Autodesk Inventor part; units mm, degrees
ref_plane "YZ Plane" through (0, 0, 0) normal (1, 0, 0) x (0, 1, 0)
ref_plane "XZ Plane" through (0, 0, 0) normal (0, 1, 0) x (-1, 0, 0)
ref_plane "XY Plane" through (0, 0, 0) normal (0, 0, 1) x (1, 0, 0)
sketch "Sketch1" plane through (0, 0, 0) normal (0, 0, 1) x (1, 0, 0)
  line L0 (0, 0) -> (51, 0)
  line L1 (51, 0) -> (51, 90)
  line L2 (51, 90) -> (0, 90)
  line L3 (0, 90) -> (0, 0)
  dimension "d0" = 51
  dimension "d1" = 90
extrude "Extrusion1" add sketch "Sketch1" along normal blind 5
sketch "Sketch2" plane through (0, 0, 5) normal (0, 0, 1) x (1, 0, 0)
  line L0 (0, 0) -> (51, 0) construction
  line L1 (25.5, 0) -> (25.5, 90) construction
  line L2 (51, 90) -> (0, 90) construction
  line L3 (51, 0) -> (51, 90) construction
  line L4 (51, 45) -> (0, 45) construction
  line L5 (25.5, 45) -> (25.5, 35) construction
  line L6 (25.5, 35) -> (18, 35) construction
  line L7 (18, 35) -> (18, 50) construction
  line L8 (18, 50) -> (33, 50) construction
  line L9 (33, 50) -> (33, 35) construction
  dimension "d23" = 10
  dimension "d24" = 7.5
  dimension "d25" = 15
  dimension "d26" = 15
sketch "Sketch3" plane through (0, 0, 0) normal (0, 0, -1) x (-1, 0, 0)
  line L0 (-51, 90) -> (0, 90)
  line L1 (-51, 90) -> (-41, 90)
  line L2 (-41, 90) -> (-41, 0)
  line L3 (0, 90) -> (-10.0159, 90)
  line L4 (-10.0159, 90) -> (-10.0159, 0)
  line L5 (0, 0) -> (-51, 0)
  line L6 (-51, 90) -> (-51, 79)
  line L7 (-51, 79) -> (0, 79)
  line L8 (-51, 0) -> (-51, 8)
  line L9 (-51, 0) -> (-51, 90)
  line L10 (-51, 8) -> (0, 8)
  line L11 (-51, 90) -> (-46, 90)
  line L12 (-51, 79) -> (-46, 79)
  line L13 (-46, 90) -> (-46, 69)
  line L14 (-10.0159, 45) -> (-4.0159, 45)
  line L15 (0, 90) -> (0, 0)
  line L16 (-41, 90) -> (-41, 48.5) construction
  line L17 (-47, 45) -> (-4.0159, 45)
  line L18 (-47, 43.5703) -> (-3.108, 43.5703)
  line L19 (-41, 90) -> (-47, 90)
  line L20 (-47, 90) -> (-47, 0)
  line L21 (-47, 0) -> (-47, 18)
  line L22 (-10.0159, 0) -> (-4.0159, 0)
  line L23 (-4.0159, 0) -> (-4.0159, 18)
  line L24 (-10.0159, 90) -> (-4.0159, 90)
  line L25 (-4.0159, 90) -> (-4.0159, 69)
  point P0 (-5, 69)
  point P1 (-46, 18)
  point P2 (-5, 18)
  point P3 (-48.5, 90)
  point P4 (-25.054, 43.5703)
  point P5 (-25.508, 45)
  point P6 (-47, 69)
  point P7 (-4.0159, 43.5703)
  dimension "d8" = 11
  dimension "d9" = 8
  dimension "d15" = 21
  dimension "d38" = 5
  dimension "d41" = 6
  dimension "d47" = 10
  dimension "d48" = 10.016
  dimension "d50" = 1.5
  dimension "d54" = 6
  dimension "d55" = 18
  dimension "d56" = 6
  dimension "d57" = 6
hole "Hole1" at (4.0159, 69, 0) at (4.0159, 43.5703, 0) at (4.0159, 18, 0) at (47, 18, 0) at (47, 43.5703, 0) at (47, 69, 0) direction (0, 0, 1) diameter 2.4 end through all counterbore diameter 4.4 counterbore depth 2
hole "Hole2" at (33, 50, 5) at (18, 50, 5) at (18, 35, 5) at (33, 35, 5) direction (0, 0, -1) diameter 2.4 end through all counterbore diameter 4.4 counterbore depth 2
chamfer "Chamfer1" distance 0.3 angle 45 4 edges at (18, 36.2, 0) (33, 36.2, 0) (18, 51.2, 0) (33, 51.2, 0)
sketch "Sketch4" plane through (0, 0, 0) normal (0, 0, -1) x (-1, 0, 0)
  circle A0 centre (-47, 69) radius 1.2
  line L0 (-47, 69) -> (-47, 57)
  circle A1 centre (-47, 18) radius 1.2
  line L1 (-47, 18) -> (-47, 30)
  circle A2 centre (-4.0159, 18) radius 1.2
  line L2 (-4.0159, 18) -> (-4.0159, 30)
  circle A3 centre (-4.0159, 69) radius 1.2
  line L3 (-4.0159, 69) -> (-4.0159, 57)
  point P0 (0, 0)
  dimension "d58" = 12
  dimension "d59" = 12
  dimension "d60" = 12
  dimension "d61" = 12
hole "Hole3" at (47, 57, 0) at (4.0159, 57, 0) at (4.0159, 30, 0) at (47, 30, 0) direction (0, 0, 1) diameter 2 end through all
chamfer "Chamfer2" distance 0.3 angle 45 4 edges at (4.0159, 29, 0) (47, 29, 0) (4.0159, 56, 0) (47, 56, 0)
properties part number "Bottom Plate" material "Steel, Carbon"
Could you check a few things on this model? Use its own coordinates, in mm. A direction names the side the tool comes from. Give positions to 0.01 mm unless a question says otherwise; leave off trailing zeros. Write each loop counter-clockwise with the first axis right and the second up, starting at its lowest first coordinate (ties: lowest second). Pieces come first, ordered by that corner, then holes. Notation, with made-up numbers: (48, 15.5) -> (85, 15.5) arc R25 cw to (85, 36.5) -> close; hole circle Ø3 at (33.25, 1.25). An arc over 180 degrees is marked (long way). Write each question's results on one line, items separated by ' | '. Start each with the question number.
Q1. I'm going to push flat-ended pins straight in: pin 1 Ø1 at (x, y) = (41.5, 35) entering from -Z; pin 2 Ø3 at (x, y) = (47, 69) entering from -Z; pin 3 Ø1.3 at (x, y) = (47, 68.5) entering from -Z. Where does each tip first touch, or does it pass through?
Q2. Suppose I cut it at A-A, the plane x = 18. List the corners of the cut face in (y, z) for me, and give its area (3 significant figures).
Q3. Suppose I cut it at B-B, the plane y = 30. List the corners of the cut face in (x, z) for me.
Q4. Which directions (+Z, -Z, +X, -X, +Y, -Y) give clear straight access to the entire face, cutting with the end or side of a thin tool? Please do faces 1 (the face through (34, 34, 3)), 2 (the face through (4.75, 17.05, 3.52)), 3 (the face through (3.36, 45.67, 1.01)).
Q5. We'd pull the mould along X, two halves only. Please class faces 4 (the face through (0, 46, 2)), 5 (the face through (32.64, 48.855, 1.631)), 6 (the face through (19, 49, 3)): +X half, -X half, draft (parallel to the pull), parting line (faces both ways), or undercut.
Q6. Suppose I cut it at C-C, the plane z = 1.15. State how many separate pieces and enclosed holes the cut face has, and give its area (3 significant figures).
Q7. I need wall thicknesses on probe 1 along X at (y, z) = (18, 2.8); probe 2 along Y at (x, z) = (47, 4.3); probe 3 along X at (y, z) = (35, 1.45). Which ranges of each line are inside material? Lowest first, please.
Outcome:
1) pin 1: z = 0 | pin 2: z = 2 | pin 3: through
2) outline: (0, 0) -> (33.5, 0) -> (33.8, 0.3) -> (33.8, 3) -> (32.8, 3) -> (32.8, 5) -> (0, 5) -> close; (36.2, 0.3) -> (36.5, 0) -> (48.5, 0) -> (48.8, 0.3) -> (48.8, 3) -> (47.8, 3) -> (47.8, 5) -> (37.2, 5) -> (37.2, 3) -> (36.2, 3) -> close; (51.2, 0.3) -> (51.5, 0) -> (90, 0) -> (90, 5) -> (52.2, 5) -> (52.2, 3) -> (51.2, 3) -> close | area: 418 mm2
3) outline: (0, 0) -> (2.72, 0) -> (3.02, 0.3) -> (3.02, 5) -> (0, 5) -> close; (5.02, 0.3) -> (5.32, 0) -> (45.7, 0) -> (46, 0.3) -> (46, 5) -> (5.02, 5) -> close; (48, 0.3) -> (48.3, 0) -> (51, 0) -> (51, 5) -> (48, 5) -> close
4) face 1: +Z | face 2: +Z, -Z | face 3: -Z
5) face 4: -X half | face 5: undercut | face 6: undercut
6) separate pieces: 1 | enclosed holes: 14 | area: 4,470 mm2
7) probe 1: 0 to 2.82, 5.22 to 45.8, 48.2 to 51 | probe 2: 0 to 16.8, 19.2 to 29, 31 to 42.37, 44.77 to 56, 58 to 67.8, 70.2 to 90 | probe 3: 0 to 16.8, 19.2 to 31.8, 34.2 to 51
